from build123d import *

# Parameters (mm, degrees)
F0_R      = 1
F1_DEPTH  = 3
F0_R_2    = 2.4
F2_DEPTH  = 7
F0_R_3    = 0.5
F3_DEPTH  = 3
F6_DEPTH  = 0.5
F7_DEPTH  = 4
F8_R      = 3
F9_R      = 1
F11_DEPTH = 0.5


with BuildPart() as f1:
    # F0 (on Front) → F1 (new body)
    with BuildSketch(Plane.XZ):
        with BuildLine():
            ThreePointArc((0, 4), (2.828427, 2.828427), (4, 0))
            ThreePointArc((4, 0), (2.828427, -2.828427), (0, -4))
            Line((0, -4), (16, -4))
            Line((16, -4), (16, 0))
            Line((16, 0), (16, 4))
            Line((16, 4), (6, 4))
            Line((6, 4), (2, 4))
            Line((2, 4), (0, 4))
        make_face()
        with Locations((11, 0)):
            Circle(F0_R, mode=Mode.SUBTRACT)
    extrude(amount=F1_DEPTH)

    # F0 (on Front) → F2 (join)
    with BuildSketch(Plane.XZ):
        with BuildLine():
            ThreePointArc((0, -4), (2.828427, -2.828427), (4, 0))
            ThreePointArc((4, 0), (2.828427, 2.828427), (0, 4))
            ThreePointArc((0, 4), (-4, 0), (0, -4))
        make_face()
        Circle(F0_R_2, mode=Mode.SUBTRACT)
    extrude(amount=F2_DEPTH)

    # F0 (on Front) → F3 (join)
    with BuildSketch(Plane.XZ):
        Circle(F0_R_2)
        Circle(F0_R_3, mode=Mode.SUBTRACT)
    extrude(amount=F3_DEPTH)

    # F5 (on Front) → F6 (cut)
    with BuildSketch(Plane.XZ):
        with BuildLine():
            Line((19.387725, -4), (19.387725, 4))
            Line((19.387725, 4), (9.719375, 4))
            ThreePointArc((9.719375, 4), (6.8, 0), (9.719375, -4))
            Line((9.719375, -4), (19.387725, -4))
        make_face()
    extrude(amount=F6_DEPTH, mode=Mode.SUBTRACT)

    # F0 (on Front) → F7 (join)
    with BuildSketch(Plane.XZ):
        Polygon((2, 6.5), (2, 4), (6, 4), (16, 4), (22, 4), (22, 6.5), align=None)
    extrude(amount=F7_DEPTH)

    # F8
    f8_edges = [f1.edges().sort_by_distance(p)[0] for p in [
        (16, -1.75, -4),
    ]]
    fillet(f8_edges, radius=F8_R)

    # F9
    f9_edges = [f1.edges().sort_by_distance(p)[0] for p in [
        (22, -2, 4),
        (22, -4, 5.25),
        (22, 0, 5.25),
        (22, -2, 6.5),
    ]]
    fillet(f9_edges, radius=F9_R)

    # F10 (on offset) → F11 (cut)
    with BuildSketch(Plane.XZ.offset(3)):
        with BuildLine():
            Line((19.387725, -4), (19.387725, 4))
            Line((19.387725, 4), (9.719375, 4))
            ThreePointArc((9.719375, 4), (6.8, 0), (9.719375, -4))
            Line((9.719375, -4), (19.387725, -4))
        make_face()
    extrude(amount=-F11_DEPTH, mode=Mode.SUBTRACT)


solid = f1.part
Geometry: final body of the model. Coordinates: model frame, mm. A direction names the side the tool comes from. Give positions to 0.01 mm unless a question says otherwise; leave off trailing zeros. Order: outer loops, then holes, each group sorted by start corner. A loop starts at its lowest first (then second) coordinate and runs counter-clockwise, first axis right, second up. Notation, with made-up numbers: (78, 76.25) -> (118, 76.25) arc R18 cw to (118, 97.25) -> close; hole circle Ø7 at (54.5, -14.75). An arc over 180 degrees is marked (long way). Answer as a JSON object with one key per item and string values.
Q1. Draft query along Z for faces 1 (the flat face through (1, -1, 4)), 2 (the flat face through (12.4, -0.5, 0.1)), 3 (the cylindrical face through (21.6, -0.2, 5.3)). Return one class per face: released by +Z, released by -Z, zero draft, split by the parting line, or undercut.
Entries:
{"face 1": "released by +Z", "face 2": "undercut", "face 3": "zero draft"}
Q2. Section D-D (x = 6.25). Output: boundary loops of the cut face in (y, z), plus the area to 3 significant figures.
Entries:
{"outline": "(-4, 4) -> (-3, 4) -> (-3, -4) -> (0, -4) -> (0, 6.5) -> (-4, 6.5) -> close", "area": "34.0 mm^2"}
Q3. Section A-A (x = 11). Output: boundary loops of the cut face in (y, z), plus the area to 3 significant figures.
Entries:
{"outline": "(-4, 4) -> (-2.5, 4) -> (-2.5, 1) -> (-0.5, 1) -> (-0.5, 4) -> (0, 4) -> (0, 6.5) -> (-4, 6.5) -> close; (-2.5, -4) -> (-0.5, -4) -> (-0.5, -1) -> (-2.5, -1) -> close", "area": "22.0 mm^2"}
Q4. Section C-C (y = -6.5). Output: boundary loops of the cut face in (x, z).
Entries:
{"outline": "circle Ø8 at (0, 0); hole circle Ø4.8 at (0, 0)"}
Q5. First-contact query: pin 1 (2 mm diameter, centred on x = 11, z = 2, fed in from +Y); pin 2 (2 mm diameter, centred on x = 9, z = 5.5, fed in from -Y); pin 3 (1 mm diameter, centred on x = 13.5, y = -5.5, fed in from +Z); pin 4 (1.4 mm diameter, centred on x = -0.5, z = 0.5, fed in from -Y). Flat tips, straight axial feed; report the tip coordinate or a pass-through.
Entries:
{"pin 1": "stops at y = -0.5", "pin 2": "stops at y = -4", "pin 3": "passes through", "pin 4": "stops at y = -3"}
Q6. Material intervals for probe 1 along Z at (x, y) = (11, -1.1); probe 2 along Z at (x, y) = (0, -2.05); probe 3 along X at (y, z) = (-4.5, 0.75), sorted ascending.
Entries:
{"probe 1": "z = -4 to -1, 1 to 6.5", "probe 2": "z = -4 to -0.5, 0.5 to 4", "probe 3": "x = -3.93 to -2.28, 2.28 to 3.93"}
Q7. Section B-B (z = 1.25). Output: boundary loops of the cut face in (x, y), plus the area to 3 significant figures.
Entries:
{"outline": "(-3.8, -7) -> (-2.05, -7) -> (-2.05, -3) -> (2.05, -3) -> (2.05, -7) -> (3.8, -7) -> (3.8, -3) -> (6.99, -3) -> (6.99, -2.5) -> (16, -2.5) -> (16, -0.5) -> (6.99, -0.5) -> (6.99, 0) -> (-3.8, 0) -> close", "area": "64.4 mm^2"}
Q8. Access query for faces 4 (the cylindrical face through (6.8, -0.2, 0.1)), 5 (the flat face through (2, -2, 5)), 6 (the cylindrical face through (1.29, -4.972, 2.024)). Directions: +Z, -Z, +X, -X, +Y, -Y. A direction counts if a zero-diameter tool reaches every point of the face in a straight line with its end or side. Return the directions, or none.
Entries:
{"face 4": "+X, +Y", "face 5": "+Z, -X, +Y, -Y", "face 6": "-Y"}
